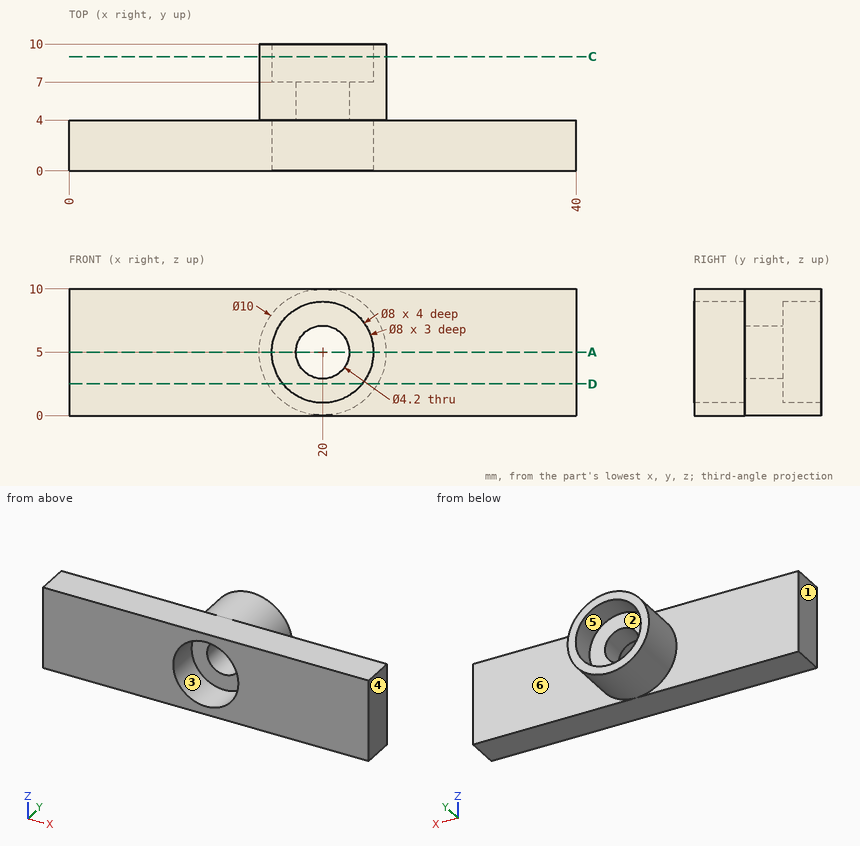
Geometry check sheet. Reference: drawing and pictorial views, mm from the part's lowest x, y, z. A direction names the side the tool comes from. Round coordinates to 2 decimals unless told otherwise and drop trailing zeros. Loops run counter-clockwise (first coordinate to the right, second up) from the corner with the lowest first, then second, coordinate; pieces in that order, holes last. Notation, with made-up numbers: (68, -17.5) - (80, -17.5) arc R10 ccw to (80, 0.5) - close; hole circle Ø2 at (48.25, -40). An arc over 180 degrees is marked (long way). Use a Markdown table: item, result. Add a question column.
1. Section check D-D, the plane z = 2.5. Record the boundary of the cut face in (x, y), plus the area to 3 significant figures.
2. Gauge pin test, flat ends, axial feed: pin 1 (4 mm diameter, centred on x = 21, z = 5.5, fed in from +Y); pin 2 (1 mm diameter, centred on x = 18, y = 3, fed in from -Z); pin 3 (4 mm diameter, centred on x = 20, z = 5, fed in from -Y); pin 4 (2.5 mm diameter, centred on x = 22, z = 5, fed in from -Y). Record the tip position at first contact, or that the pin passes through.
3. Thickness scan on probe 1 along X at (y, z) = (4.9, 5); probe 2 along Y at (x, z) = (36, 7.25); probe 3 along X at (y, z) = (2.95, 5). Record the ranges inside material, lowest first. Write a range as [from, to].
4. Section check A-A, the plane z = 5. Record the boundary of the cut face in (x, y), plus the area to 3 significant figures.
5. Access from +Z, -Z, +X, -X, +Y, -Y to the whole of each face (thin tool, end or side, straight path). Record for the marked faces 1, 2 and 3.
6. Section check C-C, the plane y = 9. Record the boundary of the cut face in (x, z), plus the area to 3 significant figures.
7. Release check for a two-part mould opening along X. For the marked faces 4, 5 and 6 record: released by +X, released by -X, zero draft, split by the parting line, or undercut.
Checks:
| question | item | result |
|---|---|---|
| 1 | outline | (0, 0) - (16.88, 0) - (16.88, 4) - (23.12, 4) - (23.12, 0) - (40, 0) - (40, 4) - (24.33, 4) - (24.33, 10) - (23.12, 10) - (23.12, 7) - (16.88, 7) - (16.88, 10) - (15.67, 10) - (15.67, 4) - (0, 4) - close |
| 1 | area | 168 mm^2 |
| 2 | pin 1 | stops at y = 7 |
| 2 | pin 2 | stops at z = 0 |
| 2 | pin 3 | passes through |
| 2 | pin 4 | stops at y = 4 |
| 3 | probe 1 | x = [15, 17.9], [22.1, 25] |
| 3 | probe 2 | y = [0, 4] |
| 3 | probe 3 | x = [0, 16], [24, 40] |
| 4 | outline | (0, 0) - (16, 0) - (16, 4) - (17.9, 4) - (17.9, 7) - (16, 7) - (16, 10) - (15, 10) - (15, 4) - (0, 4) - close; (22.1, 4) - (24, 4) - (24, 0) - (40, 0) - (40, 4) - (25, 4) - (25, 10) - (24, 10) - (24, 7) - (22.1, 7) - close |
| 4 | area | 151 mm^2 |
| 5 | face 1 | +Z, -Z, -X, +Y, -Y |
| 5 | face 2 | +Y |
| 5 | face 3 | -Y |
| 6 | outline | circle Ø10 at (20, 5); hole circle Ø8 at (20, 5) |
| 6 | area | 28.3 mm^2 |
| 7 | face 4 | released by +X |
| 7 | face 5 | undercut |
| 7 | face 6 | zero draft |
